Input: part model. Units: mm. Frame: model coordinates. A direction names the side the tool comes from. Give positions to 0.01 mm unless a question says otherwise; leave off trailing zeros. Loops run counter-clockwise (first coordinate to the right, second up) from the corner with the lowest first, then second, coordinate; pieces in that order, holes last. Notation, with made-up numbers: (9, -8.5) - (23, -8.5) arc R7 cw to (23, -1.5) - close; hole circle Ø10 at (-3, -38.75). An arc over 180 degrees is marked (long way). One line per item, written item: value.
from build123d import *

# Parameters (mm, degrees)
F1_DEPTH = 25.4
F3_DEPTH = 25.401
F5_DEPTH = 25.401
F7_DEPTH = 12.701


with BuildPart() as f1:
    # F0 (on Front) → F1 (new body)
    with BuildSketch(Plane.XZ):
        Polygon((25.4, 38.1), (0, 38.1), (0, 0), (69.85, 0), (69.85, 12.7), (25.4, 12.7), align=None)
    extrude(amount=F1_DEPTH)

    # F2 (on face) → F3 (cut, through all)
    with BuildSketch(Plane.XZ.offset(25.4)):
        with BuildLine():
            Line((6.35, 25.4), (19.05, 25.4))
            ThreePointArc((19.05, 25.4), (12.7, 31.75), (6.35, 25.4))
        make_face()
        with BuildLine():
            ThreePointArc((6.35, 25.4), (12.7, 19.05), (19.05, 25.4))
            Line((19.05, 25.4), (6.35, 25.4))
        make_face()
    extrude(amount=-F3_DEPTH, mode=Mode.SUBTRACT)

    # F4 (on face) → F5 (cut, through all)
    with BuildSketch(Plane.XZ.offset(25.4)):
        with BuildLine():
            ThreePointArc((0, 27.8021660134), (3.867394622, 34.7385435521), (11.0625794751, 38.1))
            Line((11.0625794751, 38.1), (0, 38.1))
            Line((0, 38.1), (0, 27.8021660134))
        make_face()
        with BuildLine():
            ThreePointArc((14.2694085859, 38.1), (21.6015748331, 34.6091533391), (25.4, 27.4315048009))
            Line((25.4, 27.4315048009), (25.4, 38.1))
            Line((25.4, 38.1), (14.2694085859, 38.1))
        make_face()
    extrude(amount=-F5_DEPTH, mode=Mode.SUBTRACT)

    # F6 (on face) → F7 (cut, through all)
    with BuildSketch(Plane.XY.offset(12.7)):
        with BuildLine():
            ThreePointArc((56.9451018092, -19.0466933699), (61.5670916047, -17.26199537), (63.5, -12.7))
            ThreePointArc((63.5, -12.7), (62.1319623553, -8.7626720876), (58.6173067433, -6.5218521448))
            Line((58.6173067433, -6.5218521448), (55.6826932567, -6.5218521448))
            ThreePointArc((55.6826932567, -6.5218521448), (50.8320114543, -13.3368051005), (56.9451018092, -19.0466933699))
        make_face()
        with BuildLine():
            Line((55.6826932567, -6.5218521448), (58.6173067433, -6.5218521448))
            ThreePointArc((58.6173067433, -6.5218521448), (57.15, -6.35), (55.6826932567, -6.5218521448))
        make_face()
        with BuildLine():
            Line((37.4478836052, -18.4172404403), (56.9451018092, -19.0466933699))
            ThreePointArc((56.9451018092, -19.0466933699), (50.8320114543, -13.3368051005), (55.6826932567, -6.5218521448))
            Line((55.6826932567, -6.5218521448), (36.1519202299, -6.5218521448))
            ThreePointArc((36.1519202299, -6.5218521448), (39.6665758419, -8.7626720876), (41.0346134866, -12.7))
            ThreePointArc((41.0346134866, -12.7), (40.0637056615, -16.074591438), (37.4478836052, -18.4172404403))
        make_face()
        with BuildLine():
            Line((31.5583283297, -18.2271006068), (37.4478836052, -18.4172404403))
            ThreePointArc((37.4478836052, -18.4172404403), (40.0637056615, -16.074591438), (41.0346134866, -12.7))
            ThreePointArc((41.0346134866, -12.7), (39.6665758419, -8.7626720876), (36.1519202299, -6.5218521448))
            Line((36.1519202299, -6.5218521448), (33.2173067433, -6.5218521448))
            ThreePointArc((33.2173067433, -6.5218521448), (28.3974454416, -11.8089231379), (31.5583283297, -18.2271006068))
        make_face()
        with BuildLine():
            ThreePointArc((31.5583283297, -18.2271006068), (34.4797152958, -19.0466933699), (37.4478836052, -18.4172404403))
            Line((37.4478836052, -18.4172404403), (31.5583283297, -18.2271006068))
        make_face()
        with BuildLine():
            Line((33.2173067433, -6.5218521448), (36.1519202299, -6.5218521448))
            ThreePointArc((36.1519202299, -6.5218521448), (34.6846134866, -6.35), (33.2173067433, -6.5218521448))
        make_face()
    extrude(amount=-F7_DEPTH, mode=Mode.SUBTRACT)


solid = f1.part
Item 1: Material intervals for L1, parallel to X at y = -10.75, z = 25.4; L2, parallel to Z at x = 12.7, y = -16; L3, parallel to Y at x = 32, z = 8.5, sorted ascending.
Verdict:
L1: x = 0 to 6.35, 19.05 to 25.4
L2: z = 0 to 19.05, 31.75 to 38.1
L3: y = -25.4 to -18.45, -6.95 to 0
Item 2: Draft query along X for faces 3 (the face through (27, -13, 0)), 4 (the face through (25.4, -13, 20)), 5 (the face through (3.785, -12.878, 34.661)), 6 (the face through (46, -6.522, 6)). Return one class per face: pulls with the +X half, pulls with the -X half, needs draft (parallel to the pull), parting line crosses it, or undercut.
Verdict:
face 3: needs draft
face 4: pulls with the +X half
face 5: pulls with the -X half
face 6: undercut
Item 3: Section D-D, the plane x = 53.5. Output: boundary loops of the cut face in (y, z).
Verdict:
outline: (-25.4, 0) - (-18.94, 0) - (-18.94, 12.7) - (-25.4, 12.7) - close; (-6.52, 0) - (0, 0) - (0, 12.7) - (-6.52, 12.7) - close
Item 4: Section B-B, the plane z = 7. Output: boundary loops of the cut face in (x, y), and give its area (3 significant figures).
Verdict:
outline: (0, -25.4) - (69.85, -25.4) - (69.85, 0) - (0, 0) - close; hole (36.15, -6.52) arc R6.35 ccw (long way) to (37.45, -18.42) - (56.95, -19.05) arc R6.35 ccw (long way) to (55.68, -6.52) - close
area: 1,370 mm^2
Item 5: Access query for faces 1 (the face through (14.08, -12.88, 31.6)), 2 (the face through (48, -4, 12.7)). Directions: +Z, -Z, +X, -X, +Y, -Y. A direction counts if a zero-diameter tool reaches every point of the face in a straight line with its end or side. Return the directions, or none.
Verdict:
face 1: +Y, -Y
face 2: +Z, +X, +Y, -Y
Item 6: Pin query (flat end, axial travel): P1, Ø7.5, axis at x = 50, y = -17, coming from the +Z side; P2, Ø1.5, axis at x = 21.5, y = -8, coming from the +Z side; P3, Ø12, axis at y = -19, z = 20.5, coming from the +X side. Return the tip coordinate at first contact, or that it passes through.
Verdict:
P1: stops at z = 12.7
P2: stops at z = 35.36
P3: stops at x = 25.4
Item 7: Section C-C, the plane y = -10.25. Output: boundary loops of the cut face in (x, z), and give its area (3 significant figures).
Verdict:
outline: (0, 0) - (28.83, 0) - (28.83, 12.7) - (25.4, 12.7) - (25.4, 27.43) arc R12.91 ccw to (14.27, 38.1) - (11.06, 38.1) arc R12.91 ccw to (0, 27.8) - close; (63.01, 0) - (69.85, 0) - (69.85, 12.7) - (63.01, 12.7) - close; hole circle Ø12.7 at (12.7, 25.4)
area: 907 mm^2
Item 8: Section A-A, the plane y = -21. Output: boundary loops of the cut face in (x, z), and give its area (3 significant figures).
Verdict:
outline: (0, 0) - (69.85, 0) - (69.85, 12.7) - (25.4, 12.7) - (25.4, 27.43) arc R12.91 ccw to (14.27, 38.1) - (11.06, 38.1) arc R12.91 ccw to (0, 27.8) - close; hole circle Ø12.7 at (12.7, 25.4)
area: 1,340 mm^2
